Could you check a few things on this drawing? It's one solid part, dimensions in mm from its lowest x, y, z. Give positions to 0.01 mm unless a question says otherwise; leave off trailing zeros. Loops run counter-clockwise (first coordinate to the right, second up) from the corner with the lowest first, then second, coordinate; pieces in that order, holes last. Notation, with made-up numbers: M 59.5,42 L 109.5,42 A24 ccw 109.5,57 Z; hole C 44,-8 d5. An arc over 180 degrees is marked long. Return JSON: item names as keys, results as strings. Group by question number.
1. If we mould it in two halves opening along X, with no side actions, what happens to the marked faces 1, 2 and 3? For each: +X half, -X half, draft (parallel to the pull), parting line (faces both ways), or undercut.
2. If we section it at D-D (y = 4): Write out the boundary of the cut face in (x, z).
3. For pin 1 (10 mm diameter, centred on x = 12.5, y = 5.5, fed in from -Z); pin 2 (3 mm diameter, centred on x = 23.5, z = 16.5, fed in from -Y) (1 decimal); pin 3 (10 mm diameter, centred on y = 3, z = 14, fed in from +X), each with a flat end and sliding along its axis, tell me the tip position at first contact or that it passes through.
4. If we section it at A-A (x = 6.35): Write out the boundary of the cut face in (y, z).
5. If we section it at C-C (y = 6.35): Write out the boundary of the cut face in (x, z).
6. Please list where these lines run through material, in increasing order: line 1 (X direction, y = 7.25, z = 14) (1 decimal); line 2 (Y direction, x = 6.35, z = 4.5); line 3 (X direction, y = 7, z = 16.5) (1 decimal).
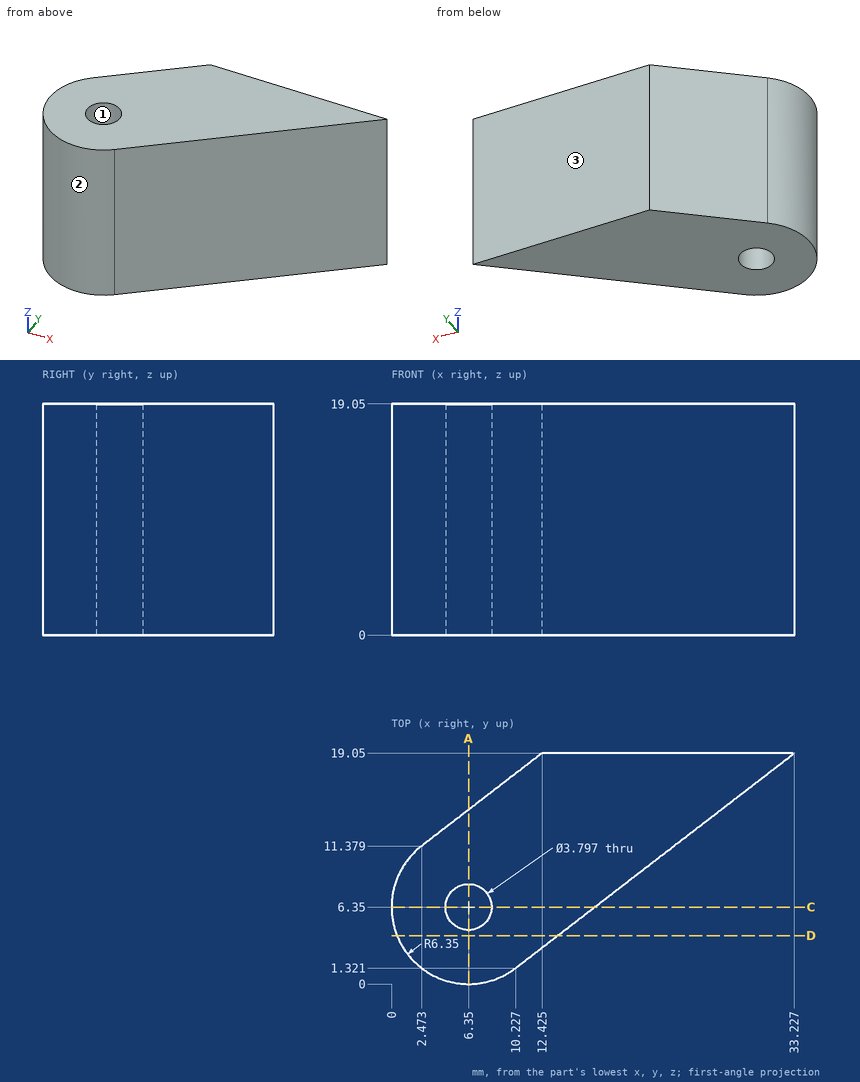
Answer:
{
 "1": {"face 1": "undercut", "face 2": "parting line", "face 3": "draft"},
 "2": {"outline": "M 0.45,0 L 13.7,0 L 13.7,19.05 L 0.45,19.05 Z"},
 "3": {"pin 1": "stops at z = 0", "pin 2": "stops at y = 10.4", "pin 3": "stops at x = 18.89"},
 "4": {"outline": "M 0,0 L 4.45,0 L 4.45,19.05 L 0,19.05 Z; M 8.25,0 L 14.37,0 L 14.37,19.05 L 8.25,19.05 Z"},
 "5": {"outline": "M 0,0 L 4.45,0 L 4.45,19.05 L 0,19.05 Z; M 8.25,0 L 16.75,0 L 16.75,19.05 L 8.25,19.05 Z"},
 "6": {"line 1": "x = 0.1 to 4.7, 8 to 17.9", "line 2": "y = 0 to 4.45, 8.25 to 14.37", "line 3": "x = 0 to 4.6, 8.1 to 17.6"}
}
